Print and shaded views of the part. All mm, measured from the part's lowest x, y and z. Give positions to 0.01 mm unless a question says otherwise; leave off trailing zeros. Loops run counter-clockwise (first coordinate to the right, second up) from the corner with the lowest first, then second, coordinate; pieces in that order, holes last. Notation, with made-up numbers: (75, 77) -> (112, 77) arc R29 ccw to (112, 105) -> close; hole circle Ø9 at (9.25, -16). An arc over 180 degrees is marked (long way). Answer as a JSON object with one key per item and string values. Group by question number.
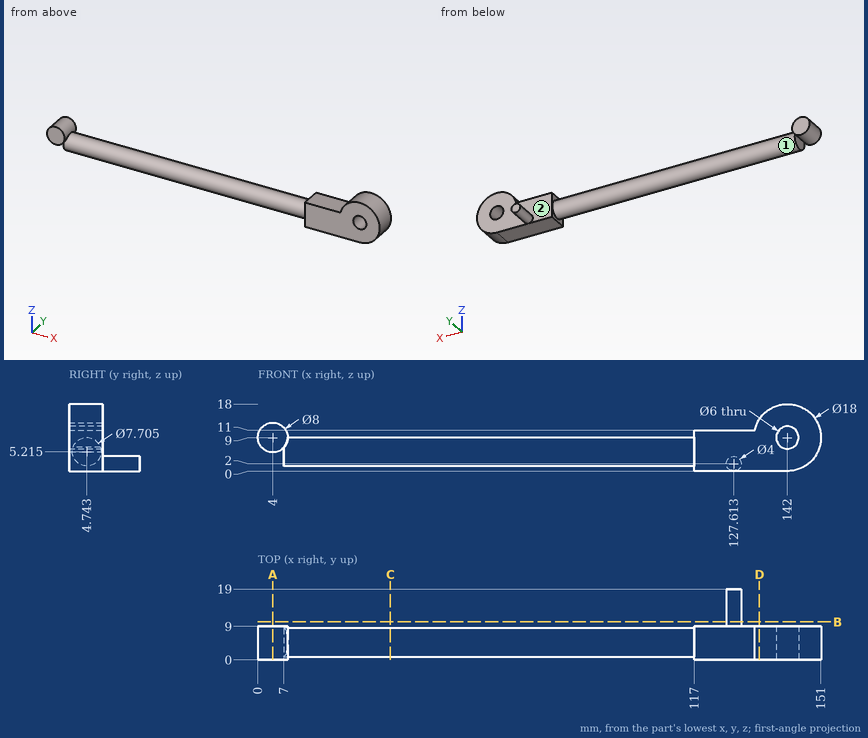
(1) Probe line 1 along X through (y, z) = (3, 9); line 2 along X through (y, z) = (5.25, 9); line 3 along X through (y, z) = (4.25, 11.25) (1 decimal). List the from-to ranges inside material, lowest first. Write a range as [from, to].
(2) Saw through at A-A on x = 4. List the corners of the cut face in (y, z), plus the area to 3 significant figures.
(3) Saw through at D-D on x = 134.5. List the corners of the cut face in (y, z) (1 decimal), plus the area to 3 significant figures.
(4) Saw through at C-C on x = 35.5. List the corners of the cut face in (y, z) (1 decimal).
(5) Saw through at B-B on y = 10.25. List the corners of the cut face in (x, z), plus the area to 3 significant figures.
(6) Pull direction X, two halves, no side cores. Call the marked faces 1 and 2: pulls with the +X half, pulls with the -X half, needs draft (parallel to the pull), parting line crosses it, or undercut.
(7) Pin check, flat tips, straight feed: pin 1 (6 mm diameter, centred on x = 45, z = 4.5, fed in from -Y); pin 2 (2 mm diameter, centred on x = 56, z = 3, fed in from -Y); pin 3 (6 mm diameter, centred on x = 109, y = 13, fed in from +Z); pin 4 (4 mm diameter, centred on x = 3.5, z = 7.5, fed in from +Y). Stop position of each tip, or through.
Calculated:
{
 "1": {"line 1": "x = [0, 8], [117, 139], [145, 151]", "line 2": "x = [0, 139], [145, 151]", "line 3": "x = [0.7, 7.3], [133.3, 140], [144, 150.7]"},
 "2": {"outline": "(0, 5) -> (9, 5) -> (9, 13) -> (0, 13) -> close", "area": "72.0 mm^2"},
 "3": {"outline": "(0, 0) -> (9, 0) -> (9, 14) -> (0, 14) -> close", "area": "126 mm^2"},
 "4": {"outline": "circle Ø7.7 at (4.7, 5.2)"},
 "5": {"outline": "circle Ø4 at (127.61, 2)", "area": "12.6 mm^2"},
 "6": {"face 1": "undercut", "face 2": "needs draft"},
 "7": {"pin 1": "stops at y = 0.89", "pin 2": "stops at y = 1.09", "pin 3": "passes through", "pin 4": "stops at y = 9"}
}
